Input: dimensioned drawing with shaded views. Units: mm. Origin: part minimum x, y, z. Round coordinates to 2 decimals unless told otherwise and drop trailing zeros. Write each loop counter-clockwise with the first axis right and the second up, starting at its lowest first coordinate (ties: lowest second). Pieces come first, ordered by that corner, then holes. Notation, with made-up numbers: (-8.5, 56.25) -> (7.5, 56.25) arc R30 ccw to (7.5, 92.25) -> close; hole circle Ø5 at (65, -32). An arc over 180 degrees is marked (long way). Return JSON: item names as keys, results as strings. Group by question number.
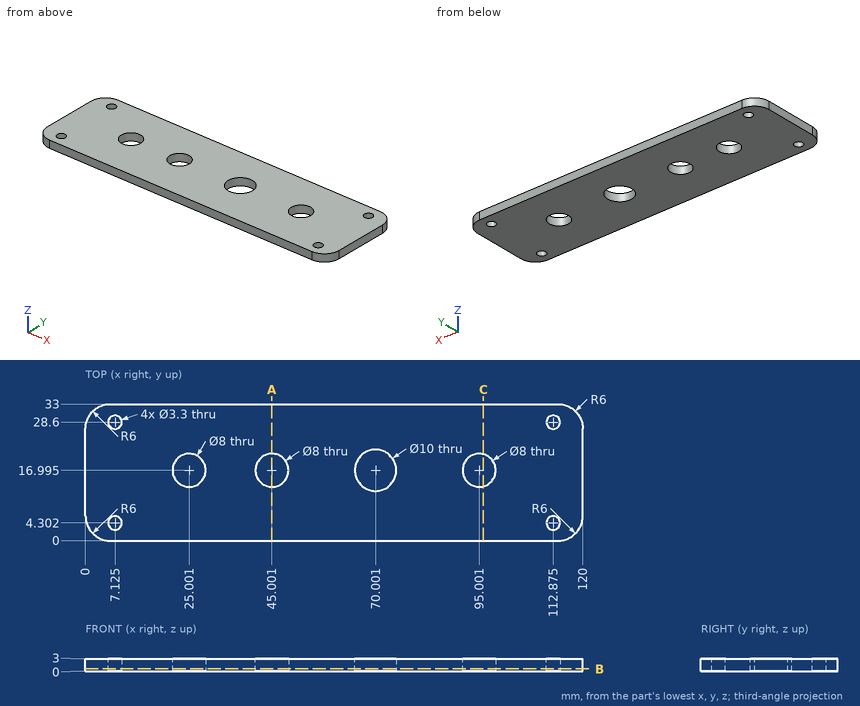
Item 1: Cut plane C-C on x = 96. Output: boundary loops of the cut face in (y, z).
Item 2: Cut plane A-A on x = 45. Output: boundary loops of the cut face in (y, z) (1 decimal).
Item 3: Cut plane B-B on z = 0.55. Give the number of separate pieces and of enclosed holes in the cut face, and give its area (3 significant figures).
Item 4: Material intervals for probe 1 along X at (y, z) = (3.5, 0.3) (1 decimal); probe 2 along X at (y, z) = (20, 1.1) (1 decimal); probe 3 along Y at (x, z) = (111.5, 0.2) (1 decimal), sorted ascending.
Here are the results:
{
 "1": {"outline": "(0, 0) -> (13.12, 0) -> (13.12, 3) -> (0, 3) -> close; (20.87, 0) -> (33, 0) -> (33, 3) -> (20.87, 3) -> close"},
 "2": {"outline": "(0, 0) -> (13, 0) -> (13, 3) -> (0, 3) -> close; (21, 0) -> (33, 0) -> (33, 3) -> (21, 3) -> close"},
 "3": {"separate pieces": "1", "enclosed holes": "8", "area": "3,670 mm^2"},
 "4": {"probe 1": "x = 0.5 to 5.7, 8.6 to 111.4, 114.3 to 119.5", "probe 2": "x = 0 to 22.4, 27.6 to 42.4, 47.6 to 66, 74 to 92.4, 97.6 to 120", "probe 3": "y = 0 to 3.4, 5.2 to 27.7, 29.5 to 33"}
}
